Here's the drawing with two shaded views (mm, measured from the low corner). I have some questions. Give positions to 0.01 mm unless a question says otherwise; leave off trailing zeros. Loops run counter-clockwise (first coordinate to the right, second up) from the corner with the lowest first, then second, coordinate; pieces in that order, holes last.
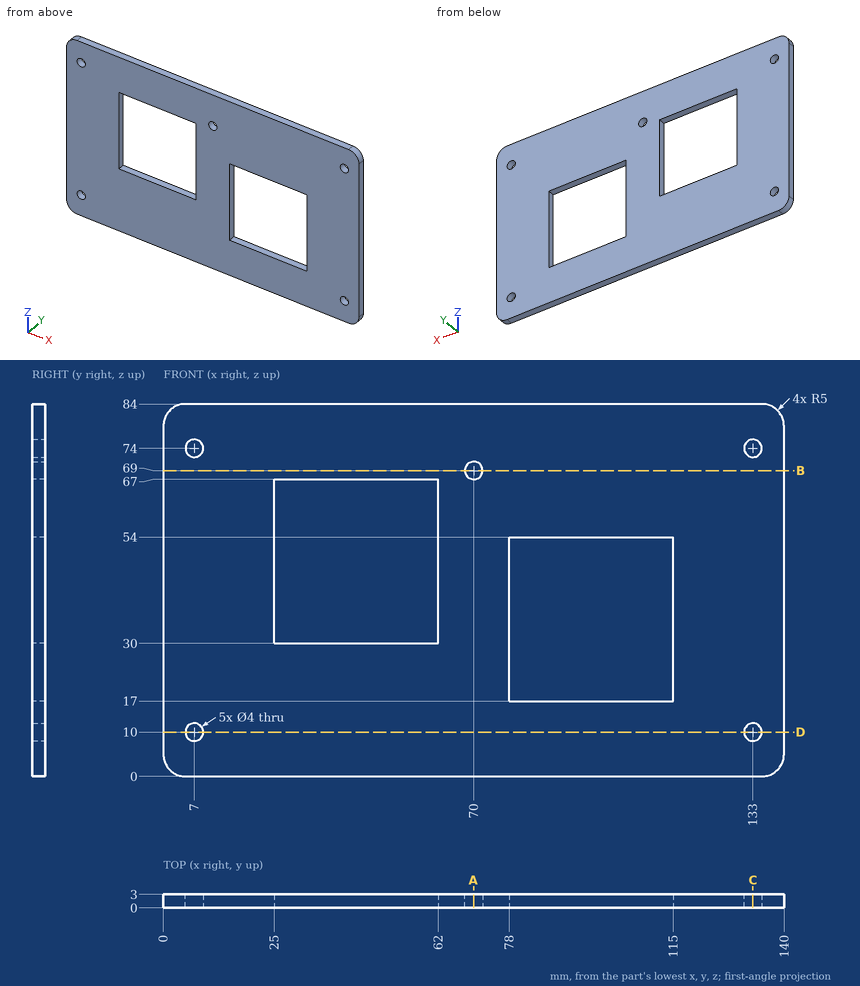
(1) Will these pins go through, and if not, where does the flat tip stop? P1, Ø0.9, axis at y = 1, z = 51, coming from the -X side; P2, Ø3, axis at x = 133, z = 10, coming from the -Y side.
Returned:
P1: stops at x = 0
P2: passes through
(2) Suppose I cut it at C-C on x = 133. List the corners of the cut face in (y, z) for me, plus the area to 3 significant figures.
Returned:
outline: (0, 0) - (3, 0) - (3, 8) - (0, 8) - close; (0, 12) - (3, 12) - (3, 72) - (0, 72) - close; (0, 76) - (3, 76) - (3, 84) - (0, 84) - close
area: 228 mm2
(3) Please list where these lines run through material, in increasing order: probe 1 along Z at (x, y) = (7, 1.8); probe 2 along X at (y, z) = (2.95, 46.5); probe 3 along Z at (x, y) = (70, 0.7).
Returned:
probe 1: z = 0 to 8, 12 to 72, 76 to 84
probe 2: x = 0 to 25, 62 to 78, 115 to 140
probe 3: z = 0 to 67, 71 to 84
(4) Suppose I cut it at A-A on x = 70. List the corners of the cut face in (y, z) for me.
Returned:
outline: (0, 0) - (3, 0) - (3, 67) - (0, 67) - close; (0, 71) - (3, 71) - (3, 84) - (0, 84) - close
(5) Suppose I cut it at B-B on z = 69. List the corners of the cut face in (x, y) for me.
Returned:
outline: (0, 0) - (68, 0) - (68, 3) - (0, 3) - close; (72, 0) - (140, 0) - (140, 3) - (72, 3) - close
(6) Suppose I cut it at D-D on z = 10. List the corners of the cut face in (x, y) for me.
Returned:
outline: (0, 0) - (5, 0) - (5, 3) - (0, 3) - close; (9, 0) - (131, 0) - (131, 3) - (9, 3) - close; (135, 0) - (140, 0) - (140, 3) - (135, 3) - close
